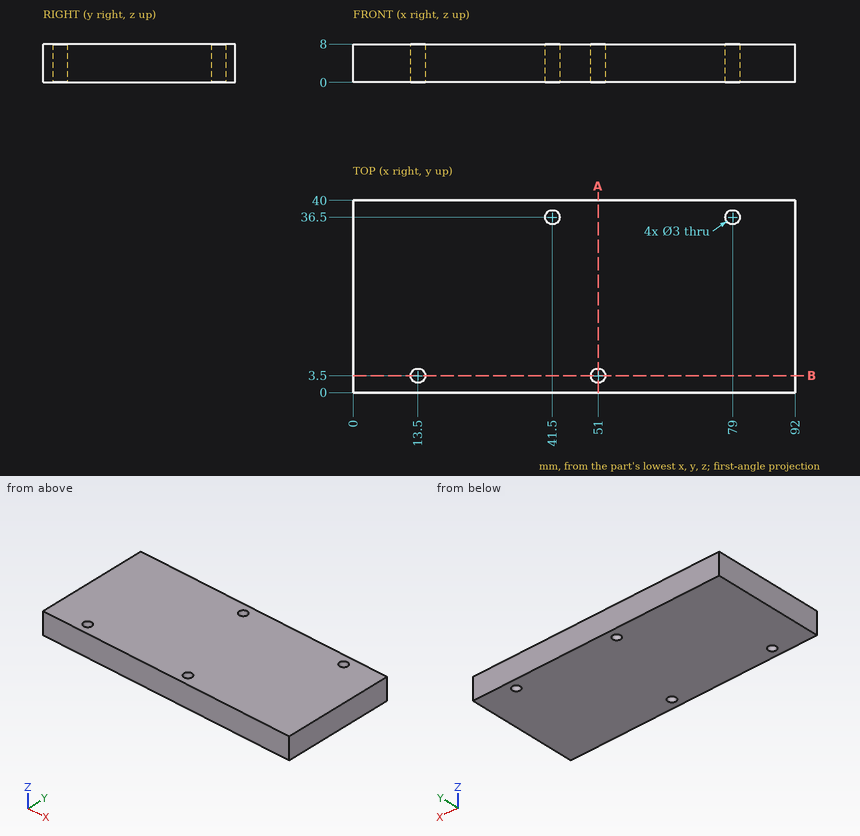
Source: three-view drawing plus pictorial views. Frame: mm from the lowest corner of the part. Coordinates: 2 decimals unless noted, no trailing zeros. Loops run counter-clockwise (first coordinate to the right, second up) from the corner with the lowest first, then second, coordinate; pieces in that order, holes last. Notation, with made-up numbers: (41, -17) - (80, -17) arc R34 ccw to (80, 14) - close; hole circle Ø4 at (-27, -29). An arc over 180 degrees is marked (long way). Answer in a Markdown table with one row per item. Add a question column.
Item 1: Section query A-A on x = 51. Return the cut outline in (y, z), then the cut area to 3 significant figures.
Item 2: Line query: line 1 along Y through (x, z) = (41.5, 3.25); line 2 along Y through (x, z) = (13.5, 3); line 3 along X through (y, z) = (36, 3). Output: solid intervals per line, ascending. Write a range as [from, to].
Item 3: Section query B-B on y = 3.5. Return the cut outline in (x, z), then the cut area to 3 significant figures.
Recorded:
| question | item | result |
|---|---|---|
| 1 | outline | (0, 0) - (2, 0) - (2, 8) - (0, 8) - close; (5, 0) - (40, 0) - (40, 8) - (5, 8) - close |
| 1 | area | 296 mm^2 |
| 2 | line 1 | [0, 35], [38, 40] |
| 2 | line 2 | [0, 2], [5, 40] |
| 2 | line 3 | [0, 40.09], [42.91, 77.59], [80.41, 92] |
| 3 | outline | (0, 0) - (12, 0) - (12, 8) - (0, 8) - close; (15, 0) - (49.5, 0) - (49.5, 8) - (15, 8) - close; (52.5, 0) - (92, 0) - (92, 8) - (52.5, 8) - close |
| 3 | area | 688 mm^2 |
